Input: part model. Units: mm. Frame: model coordinates. Face numbers are marked on the shaded views. A direction names the side the tool comes from. Coordinates: 2 decimals unless noted, no trailing zeros. Order: outer loops, then holes, each group sorted by start corner. A loop starts at its lowest first (then second) coordinate and runs counter-clockwise, first axis right, second up. Notation, with made-up numbers: M 22.25,41 L 75.25,41 A21 cw 75.25,50 Z; hole C 15.25,0 d5. An arc over 180 degrees is marked long. One line per item, written item: value.
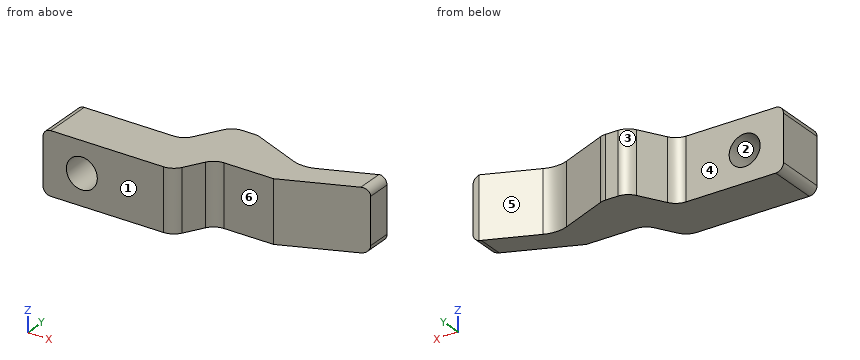
Autodesk Inventor part; units mm, degrees
ref_plane "YZ Plane" through (0, 0, 0) normal (1, 0, 0) x (0, 1, 0)
ref_plane "XZ Plane" through (0, 0, 0) normal (0, 1, 0) x (-1, 0, 0)
ref_plane "XY Plane" through (0, 0, 0) normal (0, 0, 1) x (1, 0, 0)
sketch "Sketch1" plane through (0, 0, 0) normal (0, 0, 1) x (1, 0, 0)
  line L0 (26.67, 7.62) -> (31.6865, 7.62)
  line L1 (31.6865, 7.62) -> (44.3865, 2.3595)
  line L2 (44.3865, 2.3595) -> (57.0865, 7.62)
  line L3 (42.7667, -3.81) -> (30.7028, -3.81)
  line L4 (57.0865, 7.62) -> (58.3565, 7.62)
  line L5 (58.3565, 7.62) -> (58.3565, 2.6475)
  line L6 (21.904, -0.635) -> (0, -0.635)
  line L7 (0, -0.635) -> (0, -10.795)
  line L8 (0, -10.795) -> (26.67, -10.795)
  line L9 (58.3565, 2.6475) -> (42.7667, -3.81)
  line L10 (26.67, 7.62) -> (21.904, -0.635)
  line L11 (26.67, -10.795) -> (30.7028, -3.81)
  point P0 (0, 0)
  dimension "d1" = 12.7
  dimension "d2" = 12.7
  dimension "d3" = 135
  dimension "d4" = 1.27
  dimension "d21" = 6.1695
  dimension "d22" = 11.43
  dimension "d45" = 5.08
  dimension "d48" = 7.62
  dimension "d49" = 0.635
  dimension "d50" = 10.16
  dimension "d56" = 26.67
  dimension "d57" = 120
  dimension "d58" = 120
extrude "Extrusion1" add sketch "Sketch1" along normal mid plane 12.7
sketch "Sketch3" plane through (0, -10.795, 6.35) normal (0, -1, 0) x (1, 0, 0)
  line L0 (44.3865, -12.7) -> (44.3865, 0)
  line L1 (26.67, 0) -> (0, 0)
  point P0 (0, -6.35)
  point P1 (8.001, -6.35)
  point P2 (0, -12.7)
  dimension "d26" = 36.3855
  dimension "d52" = 12.7
  dimension "d53" = 6.35
hole "Hole2" at (8.001, -10.795, 0) direction (0, 1, 0) diameter 6.3754 end through all
fillet "Fillet3" radius 6.35 1 edges at (44.3865, 2.3595, 0)
chamfer "Chamfer2" [suppressed]
fillet "Fillet5" [suppressed]
fillet "Fillet1" radius 1.5875 4 edges at (58.3565, 5.1337, 6.35) (58.3565, 5.1337, -6.35) (0, -5.715, -6.35) (0, -5.715, 6.35)
fillet "Fillet6" radius 3.175 5 edges at (21.904, -0.635, 0) (26.67, 7.62, 0) (31.6865, 7.62, 0) (26.67, -10.795, 0) (30.7028, -3.81, 0)
properties part number "J002865" material "ALUMINUM, 6061-T651"
(1) Ray query, line 1 (Z direction, x = 10, y = -1.5); line 2 (Y direction, x = 18, z = 0) (3 decimals); line 3 (X direction, y = -3.75, z = 0). Return the intervals inside material, ascending. Write a range as from..to.
Data:
line 1: z = -6.35..-2.48, 2.48..6.35
line 2: y = -10.795..-0.635
line 3: x = 0..4.81, 11.19..42.91
(2) Draft query along X for the marked faces 1, 2 and 3. Return one class per face: released by +X, released by -X, zero draft, split by the parting line, or undercut.
Data:
face 1: zero draft
face 2: undercut
face 3: released by -X
(3) Cut plane D-D on x = 13. Output: boundary loops of the cut face in (y, z) (3 decimals).
Data:
outline: M -10.795,-6.35 L -0.635,-6.35 L -0.635,6.35 L -10.795,6.35 Z
(4) First-contact query: pin 1 (1 mm diameter, centred on y = 1.5, z = -4, fed in from -X); pin 2 (3 mm diameter, centred on x = 38.5, z = 2, fed in from -Y); pin 3 (4 mm diameter, centred on y = 4, z = 4.5, fed in from -X); pin 4 (5.5 mm diameter, centred on x = 8.001, z = 0, fed in from +Y). Flat tips, straight axial feed; report the tip coordinate or a pass-through.
Data:
pin 1: stops at x = 22.85
pin 2: stops at y = -3.81
pin 3: stops at x = 23.43
pin 4: passes through
(5) Access query for the marked faces 4, 5 and 6. Directions: +Z, -Z, +X, -X, +Y, -Y. A direction counts if a zero-diameter tool reaches every point of the face in a straight line with its end or side. Return the directions, or none.
Data:
face 4: +Z, -Z, -X, +Y
face 5: +Z, -Z, +Y
face 6: +Z, -Z, +X, -Y
